Autodesk Fusion 360 part; units mm, degrees
sketch "Esboço1" plane through (0, 0, 0) normal (0, 0, 1) x (1, 0, 0) in component "Case"
sketch "Esboço1 (2)" plane through (0, 0, 0) normal (0, 0, 1) x (1, 0, 0) in component "Component"
  line L0 (-33.5931, -47.7327) -> (13.2718, -47.7327)
  line L1 (13.2718, -47.7327) -> (13.2718, 52.2673)
  line L2 (13.2718, 52.2673) -> (-33.5931, 52.2673)
  line L3 (-33.5931, 52.2673) -> (-33.5931, -47.7327)
  line L4 (-40, 60) -> (20, 60)
  line L5 (20, 60) -> (20, -55)
  line L6 (20, -55) -> (-40, -55)
  line L7 (-40, -55) -> (-40, 60)
  circle A0 centre (-35, -50) radius 1.7
  circle A1 centre (15, -50) radius 1.7
  circle A2 centre (-35, 55) radius 1.7
  circle A3 centre (15, 55) radius 1.7
  dimension "d1" = 100
  dimension "d2" = 46.8649
  dimension "d5" = 5
  dimension "d6" = 5
  dimension "d7" = 5
  dimension "d8" = 5
  dimension "d9" = 5
  dimension "d10" = 5
  dimension "d11" = 5
  dimension "d12" = 5
  dimension "d13" = 60
  dimension "d14" = 115
extrude "Extrusão1" add sketch "Esboço1 (2)" along normal blind 9.9 contours A0 | A1 | A2 | A3 makes body 1 at (-35.7756, -48.4872, 6.6) makes body 2 at (-35.7756, 56.5128, 6.6) makes body 3 at (16.5665, -49.3397, 6.6) makes body 4 at (16.5665, 55.6603, 6.6) in component "Component"
extrude "Extrusão2" add sketch "Esboço1 (2)" along normal blind 13 bodies 1 2 3 4 in component "Component"
extrude "Extrusão3" add sketch "Esboço1 (2)" along normal blind 3 contours L0 L1 L2 L3 bodies 1 in component "Component"
sketch "Esboço2" plane through (0, 0, 13) normal (0, 0, 1) x (-1, 0, 0) in component "Component"
  circle A0 centre (-15, -55) radius 1.7
  line L0 (33.5931, 47.7327) -> (33.5931, -52.2673)
  line L1 (33.5931, -52.2673) -> (-13.2718, -52.2673)
  line L2 (-13.2718, -52.2673) -> (-13.2718, 47.7327)
  line L3 (-13.2718, 47.7327) -> (33.5931, 47.7327)
  circle A1 centre (35, 50) radius 1.7
  circle A2 centre (-15, 50) radius 1.7
  circle A3 centre (35, -55) radius 1.7
  line L4 (40, 55) -> (-20, 55)
  line L5 (-20, 55) -> (-20, -60)
  line L6 (-20, -60) -> (40, -60)
  line L7 (40, -60) -> (40, 55)
  line L8 (15.0931, -60) -> (6.2282, -60)
  line L9 (6.2282, -60) -> (6.2282, -52.2673)
  line L10 (6.2282, -52.2673) -> (15.0931, -52.2673)
  line L11 (15.0931, -52.2673) -> (15.0931, -60)
  dimension "d21" = 18.5
  dimension "d22" = 19.5
extrude "Extrusão4" cut sketch "Esboço2" against normal blind 7.5 contours L1 L6 L8 L9 L10 L11 bodies 1 in component "Component"
fillet "Arredondamento1" radius 5 1 edges at (20, -55, 6.5) on bodies 1 in component "Component"
fillet "Arredondamento2" radius 5 1 edges at (-40, -55, 6.5) on bodies 1 in component "Component"
fillet "Arredondamento3" radius 5 1 edges at (-40, 60, 6.5) on bodies 1 in component "Component"
fillet "Arredondamento4" radius 5 1 edges at (20, 60, 6.5) on bodies 1 in component "Component"
component "Case" placed x (1, 0, 0) y (0, 1, 0) z (0, 0, 1) at (0, 0, 0)
component "Component" placed x (1, 0, 0) y (0, 1, 0) z (0, 0, 1) at (0, 0, 0) in component "Case"
Geometry check sheet. Reference: the model listing, model coordinates, mm. A direction names the side the tool comes from. Give positions to 0.01 mm unless a question says otherwise; leave off trailing zeros. Write each loop counter-clockwise with the first axis right and the second up, starting at its lowest first coordinate (ties: lowest second). Pieces come first, ordered by that corner, then holes. Notation, with made-up numbers: M -24,25.5 L 16,25.5 A8 cw 16,38.5 Z; hole C 50.5,85.25 d11. An arc over 180 degrees is marked long. Answer as CSV lines item,"result". Start each with the question number.
Q1. Go/stop test with flat-tipped pins: pin 1 (5.5 mm diameter, centred on x = 15, y = -50, fed in from +Z); pin 2 (23.5 mm diameter, centred on x = -14, y = 8, fed in from +Z); pin 3 (1 mm diameter, centred on x = 15.5, y = 55, fed in from +Z). Record where each tip stops, or that it passes through.
Q2. Section check C-C, the plane z = 8.25. Record the cut outline in (x, y).
Q3. Release check for a two-part mould opening along Y. For faces 4 (the face through (18, -54, 7)), 5 (the face through (-10, -47.733, 8)), 6 (the face through (-33.593, 3, 8)), 7 (the face through (20, 3, 6)) record: pulls with the +Y half, pulls with the -Y half, needs draft (parallel to the pull), parting line crosses it, or undercut.
Q4. Material ranges on L1, parallel to Y at x = -35, z = 11.25; L2, parallel to X at y = 24, z = 10; L3, parallel to Y at x = -18.5, z = 4, recorded low to high.
Q5. Section check A-A, the plane x = -21.5. Record the cut outline in (y, z).
Q6. Section check B-B, the plane y = -15. Record the cut outline in (x, z).
Q7. Tool access check on faces 1 (the face through (-39, -53, 7)), 2 (the face through (-11, 56, 5.5)), 3 (the face through (-10, 3, 3)). Record the directions out of +Z, -Z, +X, -X, +Y, -Y that give a thin tool (end or side, any length) a straight path to the whole face; none if there is none.
Geometry says:
1,pin 1,"z = 13"
1,pin 2,"z = 3"
1,pin 3,"z = 9.9"
2,outline,"M -40,-50 A5 ccw -35,-55 L 15,-55 A5 ccw 20,-50 L 20,55 A5 ccw 15,60 L -6.23,60 L -6.23,52.27 L 13.27,52.27 L 13.27,-47.73 L -33.59,-47.73 L -33.59,52.27 L -15.09,52.27 L -15.09,60 L -35,60 A5 ccw -40,55 Z"
3,face 4,"pulls with the -Y half"
3,face 5,"undercut"
3,face 6,"undercut"
3,face 7,"needs draft"
4,L1,"-55 to -51.7, -48.3 to 53.3, 56.7 to 60"
4,L2,"-40 to -33.59, 13.27 to 20"
4,L3,"-55 to -47.73, 52.27 to 60"
5,outline,"M -55,0 L 60,0 L 60,13 L 52.27,13 L 52.27,3 L -47.73,3 L -47.73,13 L -55,13 Z"
6,outline,"M -40,0 L 20,0 L 20,13 L 13.27,13 L 13.27,3 L -33.59,3 L -33.59,13 L -40,13 Z"
7,face 1,"+Z, -Z, -X, -Y"
7,face 2,"+Z, +Y"
7,face 3,"+Z"
